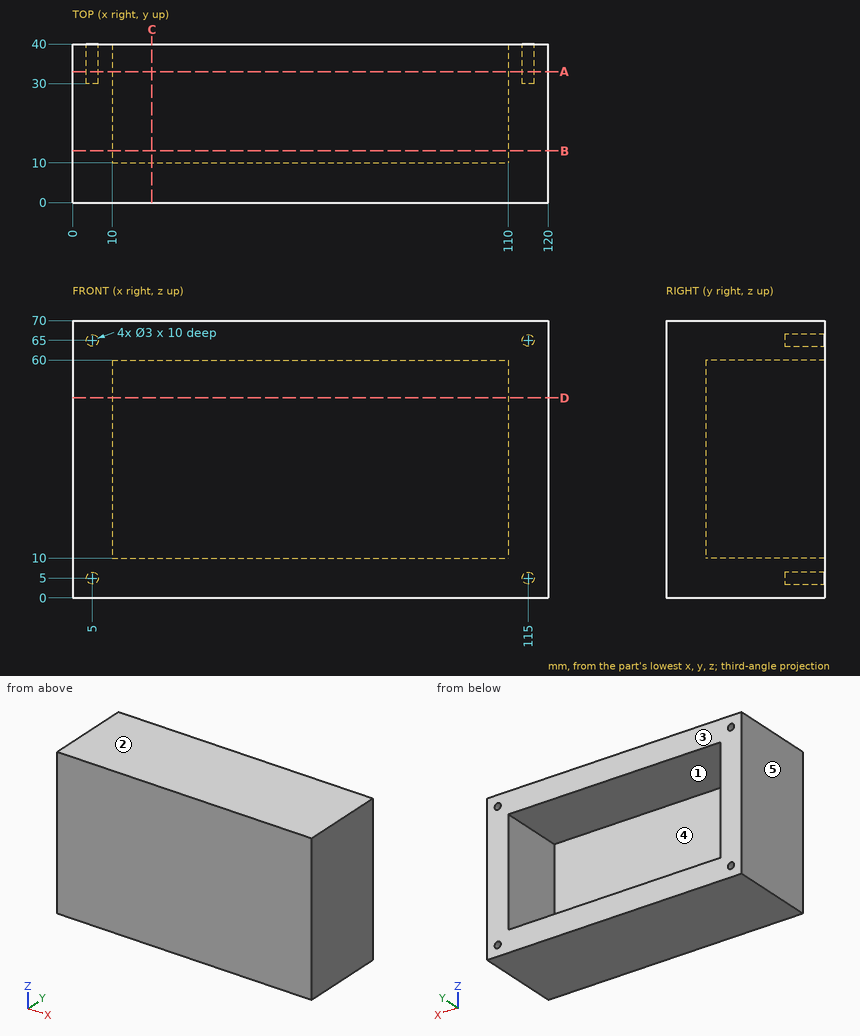
Geometry check sheet. Reference: drawing and pictorial views, mm from the part's lowest x, y, z. A direction names the side the tool comes from. Coordinates: 2 decimals unless noted, no trailing zeros. Loops run counter-clockwise (first coordinate to the right, second up) from the corner with the lowest first, then second, coordinate; pieces in that order, holes last. Notation, with made-up numbers: (38, 9.25) - (71, 9.25) arc R14 cw to (71, 35.25) - close; hole circle Ø7 at (52, -34). An arc over 180 degrees is marked (long way). Return JSON: item names as keys, results as strings.
1. Section check D-D, the plane z = 50.5. Record the boundary of the cut face in (x, y), then the cut area to 3 significant figures.
Established:
{"outline": "(0, 0) - (120, 0) - (120, 40) - (110, 40) - (110, 10) - (10, 10) - (10, 40) - (0, 40) - close", "area": "1,800 mm2"}
2. Thickness scan on L1, parallel to X at y = 34, z = 65; L2, parallel to Z at x = 115, y = 33; L3, parallel to X at y = 27, z = 33. Record the ranges inside material, lowest first.
Established:
{"L1": "x = 0 to 3.5, 6.5 to 113.5, 116.5 to 120", "L2": "z = 0 to 3.5, 6.5 to 63.5, 66.5 to 70", "L3": "x = 0 to 10, 110 to 120"}
3. Go/stop test with flat-tipped pins: pin 1 (2.5 mm diameter, centred on x = 115, z = 65, fed in from +Y); pin 2 (2 mm diameter, centred on x = 27, z = 39.5, fed in from +Y). Record where each tip stops, or that it passes through.
Established:
{"pin 1": "stops at y = 30", "pin 2": "stops at y = 10"}
4. Section check A-A, the plane y = 33. Record the boundary of the cut face in (x, z), then the cut area to 3 significant figures.
Established:
{"outline": "(0, 0) - (120, 0) - (120, 70) - (0, 70) - close; hole circle Ø3 at (5, 5); hole circle Ø3 at (5, 65); hole (10, 10) - (110, 10) - (110, 60) - (10, 60) - close; hole circle Ø3 at (115, 5); hole circle Ø3 at (115, 65)", "area": "3,370 mm2"}
5. Mould release check, pull along X, two halves, no side actions. Record for the marked faces 3, 4 and 5: +X half, -X half, draft (parallel to the pull), parting line (faces both ways), or undercut.
Established:
{"face 3": "draft", "face 4": "undercut", "face 5": "-X half"}
6. Section check B-B, the plane y = 13. Record the boundary of the cut face in (x, z).
Established:
{"outline": "(0, 0) - (120, 0) - (120, 70) - (0, 70) - close; hole (10, 10) - (110, 10) - (110, 60) - (10, 60) - close"}
7. Tool access check on the marked faces 1 and 2. Record the directions out of +Z, -Z, +X, -X, +Y, -Y that give a thin tool (end or side, any length) a straight path to the whole face; none if there is none.
Established:
{"face 1": "+Y", "face 2": "+Z, +X, -X, +Y, -Y"}
8. Section check C-C, the plane x = 20. Record the boundary of the cut face in (y, z), then the cut area to 3 significant figures.
Established:
{"outline": "(0, 0) - (40, 0) - (40, 10) - (10, 10) - (10, 60) - (40, 60) - (40, 70) - (0, 70) - close", "area": "1,300 mm2"}
